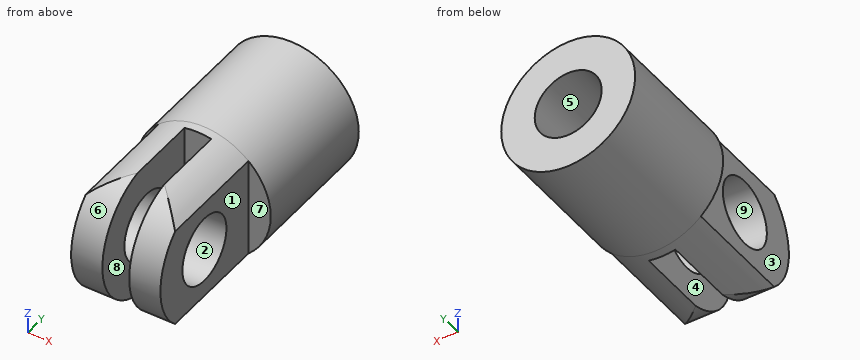
```python
from build123d import *

# Parameters (mm, degrees)
F0_R      = 9.525
F0_R_2    = 4.7625
F1_DEPTH  = 19.05
F3_DEPTH  = 19.05
F4_R      = 4.7625
F5_DEPTH  = 15.876
F7_DEPTH  = 15.876
F8_W      = 3.81
F8_H      = 20.32
F9_DEPTH  = 9.526
F10_DEPTH = 9.526


with BuildPart() as f1:
    # F0 (on Front) → F1 (new body)
    with BuildSketch(Plane.XZ):
        Circle(F0_R)
        Circle(F0_R_2, mode=Mode.SUBTRACT)
    extrude(amount=F1_DEPTH)

    # F2 (on face) → F3 (join)
    with BuildSketch(Plane.XZ.offset(19.05)):
        with BuildLine():
            Line((-6.35, 7.099516), (-6.35, -7.099516))
            ThreePointArc((-6.35, -7.099516), (0, -9.525), (6.35, -7.099516))
            Line((6.35, -7.099516), (6.35, 7.099516))
            ThreePointArc((6.35, 7.099516), (0, 9.525), (-6.35, 7.099516))
        make_face()
    extrude(amount=F3_DEPTH)

    # F4 (on face) → F5 (cut, through all)
    with BuildSketch(Plane(origin=(-6.35, 0, 0), x_dir=(0, -1, 0), z_dir=(-1, 0, 0))):
        with Locations((28.575, 0)):
            Circle(F4_R)
    extrude(amount=-F5_DEPTH, mode=Mode.SUBTRACT)

    # F6 (on face) → F7 (cut, through all)
    with BuildSketch(Plane.YZ.offset(6.35)):
        with BuildLine():
            ThreePointArc((-28.854043, -9.520912), (-38.1, 0), (-28.854043, 9.520912))
            Line((-28.854043, 9.520912), (-28.854043, 11.027435))
            Line((-28.854043, 11.027435), (-38.735, 11.027435))
            Line((-38.735, 11.027435), (-38.735, 9.520912))
            Line((-38.735, 9.520912), (-38.735, -9.520912))
            Line((-38.735, -9.520912), (-38.735, -10.820097))
            Line((-38.735, -10.820097), (-28.854043, -10.820097))
            Line((-28.854043, -10.820097), (-28.854043, -9.520912))
        make_face()
    extrude(amount=-F7_DEPTH, mode=Mode.SUBTRACT)

    # F8 (on Top) → F9 (cut, through all)
    with BuildSketch(Plane.XY):
        with Locations((0, -30.48)):
            Rectangle(F8_W, F8_H)
    extrude(amount=-F9_DEPTH, mode=Mode.SUBTRACT)

    # F8 (on Top) → F10 (cut, through all)
    with BuildSketch(Plane.XY):
        with Locations((0, -30.48)):
            Rectangle(F8_W, F8_H)
    extrude(amount=F10_DEPTH, mode=Mode.SUBTRACT)


solid = f1.part
```
Source: CAD feature listing. Evaluate the final solid. Frame: model axes, mm. Face numbers are marked on the shaded views. A direction names the side the tool comes from. Give positions to 0.01 mm unless a question says otherwise; leave off trailing zeros. Loops run counter-clockwise (first coordinate to the right, second up) from the corner with the lowest first, then second, coordinate; pieces in that order, holes last. Notation, with made-up numbers: (33, 5.5) -> (86, 5.5) arc R24 ccw to (86, 26.5) -> close; hole circle Ø5 at (48.5, 83.5). An arc over 180 degrees is marked (long way). Put each result on its own line as item: value. Start each with the question number.
1) Cut plane B-B (z = 0). State how many separate pieces and enclosed holes the cut face has, then the cut area to 3 significant figures.
2) Reachability of the marked faces 5, 6, 7, 8 and 9 from +Z, -Z, +X, -X, +Y, -Y: full face, straight path, thin tool, end or side. Return the list, or none.
3) Material intervals for probe 1 along Y at (x, z) = (-3.5, -0.25); probe 2 along Y at (x, z) = (4.8, 0); probe 3 along X at (y, z) = (-27.5, -6) (3 decimals), sorted ascending.
4) Contact query for flat-ended pins moving along their axis: P1, Ø9, axis at y = -33, z = 4, coming from the -X side; P2, Ø11, axis at x = 0, z = 0, coming from the +Y side; P3, Ø5, axis at y = -15, z = -6, coming from the +X side; P4, Ø3, axis at x = 0.5, z = -2.5, coming from the -Y side. Output: stop coordinate, or through.
5) Cut plane A-A (y = -21). Return loops of the section in (x, z) (3 decimals), then the cut area to 3 significant figures.
6) Draft query along X for the marked faces 1, 2, 3 and 4. Return one class per face: released by +X, released by -X, zero draft, split by the parting line, or undercut.
7) Cut plane D-D (y = -27.5). Return loops of the section in (x, z) (3 decimals), then the cut area to 3 significant figures.
Results are:
1. separate pieces: 3
1. enclosed holes: 0
1. area: 271 mm2
2. face 5: +Y
2. face 6: +X, -X, -Y
2. face 7: +Z, -Z, +X, -Y
2. face 8: +Z, -Z, -Y
2. face 9: +X, -X
3. probe 1: y = -38.1 to -33.33, -23.82 to -19.05
3. probe 2: y = -38.1 to -33.34, -23.81 to 0
3. probe 3: x = -6.35 to -1.905, 1.905 to 6.35
4. P1: stops at x = -6.35
4. P2: stops at y = 0
4. P3: stops at x = 8.86
4. P4: stops at y = -37.89
5. outline: (-6.35, -7.1) arc R9.525 ccw to (-1.905, -9.333) -> (-1.905, 9.333) arc R9.525 ccw to (-6.35, 7.1) -> close; (1.905, -9.333) arc R9.525 ccw to (6.35, -7.1) -> (6.35, 7.1) arc R9.525 ccw to (1.905, 9.333) -> close
5. area: 150 mm2
6. face 1: released by +X
6. face 2: zero draft
6. face 3: released by -X
6. face 4: undercut
7. outline: (-6.35, -7.1) arc R9.525 ccw to (-1.905, -9.333) -> (-1.905, -4.64) -> (-6.35, -4.64) -> close; (-6.35, 4.64) -> (-1.905, 4.64) -> (-1.905, 9.333) arc R9.525 ccw to (-6.35, 7.1) -> close; (1.905, -9.333) arc R9.525 ccw to (6.35, -7.1) -> (6.35, -4.64) -> (1.905, -4.64) -> close; (1.905, 4.64) -> (6.35, 4.64) -> (6.35, 7.1) arc R9.525 ccw to (1.905, 9.333) -> close
7. area: 68.0 mm2
